from build123d import *

# Parameters (mm, degrees)
SKETCH2_W           = 50.8
SKETCH2_H           = 49.53
BOSS_EXTRUDE1_DEPTH = 1.6
SKETCH3_R           = 1.4
CUT_EXTRUDE1_DEPTH  = 1.6


with BuildPart() as part:
    # Sketch2 → Boss-Extrude1 (new body)
    with BuildSketch(Plane(origin=(0, 0, 0), x_dir=(1, 0, 0), z_dir=(0, 1, 0))):
        Rectangle(SKETCH2_W, SKETCH2_H)
    extrude(amount=BOSS_EXTRUDE1_DEPTH)

    # Sketch3 → Cut-Extrude1 (cut)
    with BuildSketch(Plane(origin=(0, 1.6, 0), x_dir=(1, 0, 0), z_dir=(0, 1, 0))):
        with Locations((-22.86, 22.225)):
            Circle(SKETCH3_R)
        with Locations((22.86, 22.225)):
            Circle(SKETCH3_R)
        with Locations((-22.86, -22.225)):
            Circle(SKETCH3_R)
    extrude(amount=-CUT_EXTRUDE1_DEPTH, mode=Mode.SUBTRACT)


solid = part.part
Verification items for the finished model (mm, model axes). Give positions to 0.01 mm unless a question says otherwise; leave off trailing zeros. Write each loop counter-clockwise with the first axis right and the second up, starting at its lowest first coordinate (ties: lowest second). Pieces come first, ordered by that corner, then holes. Notation, with made-up numbers: (78, 80.25) - (96, 80.25) arc R12 cw to (96, 99.25) - close; hole circle Ø4 at (-22, 48). An arc over 180 degrees is marked (long way). Answer as CSV lines item,"result". Start each with the question number.
1. Thickness scan on line 1 (Z direction, x = -22.86, y = 1.2) (3 decimals); line 2 (Z direction, x = 22.86, y = 1) (3 decimals); line 3 (X direction, y = 1.4, z = 23). Record the ranges inside material, lowest first.
2. Sectioned sample at B-B (x = 22.86). Record the boundary of the cut face in (y, z) (3 decimals).
3. Draft check along X on faces 1 (the face through (25.4, 1, 0)), 2 (the face through (24.195, 0.811, -22.646)), 3 (the face through (0, 1.6, 0)). Enter one of: pulls with the +X half, pulls with the -X half, needs draft (parallel to the pull), parting line crosses it, or undercut.
4. Sectioned sample at A-A (x = -22.86). Record the boundary of the cut face in (y, z) (3 decimals), then the cut area to 3 significant figures.
Derived:
1,line 1,"-24.765 to -23.625, -20.825 to 20.825, 23.625 to 24.765"
1,line 2,"-24.765 to -23.625, -20.825 to 24.765"
1,line 3,"-25.4 to -24.03, -21.69 to 25.4"
2,outline,"(0, -24.765) - (1.6, -24.765) - (1.6, -23.625) - (0, -23.625) - close; (0, -20.825) - (1.6, -20.825) - (1.6, 24.765) - (0, 24.765) - close"
3,face 1,"pulls with the +X half"
3,face 2,"undercut"
3,face 3,"needs draft"
4,outline,"(0, -24.765) - (1.6, -24.765) - (1.6, -23.625) - (0, -23.625) - close; (0, -20.825) - (1.6, -20.825) - (1.6, 20.825) - (0, 20.825) - close; (0, 23.625) - (1.6, 23.625) - (1.6, 24.765) - (0, 24.765) - close"
4,area,"70.3 mm²"
